Input: part model. Units: mm. Frame: model coordinates. A direction names the side the tool comes from. Coordinates: 2 decimals unless noted, no trailing zeros. Loops run counter-clockwise (first coordinate to the right, second up) from the corner with the lowest first, then second, coordinate; pieces in that order, holes last. Notation, with made-up numbers: (41, 31.25) -> (81, 31.25) arc R36 cw to (81, 67.25) -> close; hole circle Ø8 at (78.25, 70). An arc over 180 degrees is marked (long way). Put each result on its own line as item: value. Start each with the question number.
1) Material intervals for L1, parallel to X at y = 25, z = 58; L2, parallel to Y at x = 6, z = 56 (3 decimals); L3, parallel to X at y = -9.5, z = -5, sorted ascending.
2) Pull-direction query (X, two-part tool) for faces 1 (the flat face through (0, 11, 60.325)), 2 (the cylindrical face through (28.465, 14.972, 26.433)), 3 (the flat face through (-31.75, -1, 2)); classes: pulls with the +X half, pulls with the -X half, needs draft (parallel to the pull), parting line crosses it, or undercut.
3) Set-up query: faces 4 (the flat face through (-27, 15.875, -51)), 5 (the cylindrical face through (-28.63, 14.94, 26.3)), 6 (the cylindrical face through (0.493, 1.87, -52.925)). Return all of +Z, -Z, +X, -X, +Y, -Y with unobstructed straight access to the full face (end or side cutting, diameter ignored); none if empty.
4) Cut plane A-A (x = -6). Return the cut outline in (y, z) (3 decimals), plus the area to 3 significant figures.
5) Cut plane B-B (z = 36). Return the cut outline in (x, y) (3 decimals), plus the area to 3 significant figures.
6) Contact query for flat-ended pins moving along their axis: P1, Ø8, axis at x = -6.35, y = 25.4, coming from the -Z side (3 decimals); P2, Ø19, axis at x = 3, y = 26.5, coming from the -Z side; P3, Ø4, axis at x = 6.35, y = 25.4, coming from the +Z side; P4, Ø12, axis at x = -27.5, z = -47, coming from the +Y side (3 decimals). Output: stop coordinate, or through.
7) Cut plane D-D (y = 9). State how many separate pieces and enclosed holes the cut face has, plus the area to 3 significant figures.
8) Cut plane C-C (x = -28). Return the cut outline in (y, z) (1 decimal), plus the area to 3 significant figures.
from build123d import *

# Parameters (mm, degrees)
SKETCH1_W               = 107.95
SKETCH1_H               = 31.75
BOSS_EXTRUDE1_DEPTH     = 31.75
SKETCH3_W               = 63.5
SKETCH3_H               = 76.2
SKETCH3_R               = 3.429
BOSS_EXTRUDE2_DEPTH     = 6.35
FILLET1_R               = 5.08
CUT_EXTRUDE1_DEPTH      = 119.79762203
CUT_EXTRUDE1_DEPTH_BACK = 119.79762203
SKETCH4_W               = 78.111463513
SKETCH4_H               = 26.600111828


with BuildPart() as part:
    # Sketch1 → Boss-Extrude1 (new, symmetric)
    with BuildSketch(Plane(origin=(0, 0, 0), x_dir=(0, 0, -1), z_dir=(1, 0, 0))):
        Rectangle(SKETCH1_W, SKETCH1_H)
    extrude(amount=BOSS_EXTRUDE1_DEPTH, both=True)

    # Sketch2 → Cut-Revolve1 (revolve, cut)
    with BuildSketch(Plane(origin=(0, 0, 0), x_dir=(0, 0, -1), z_dir=(1, 0, 0))):
        Polygon((30.787113889, -1.024256513), (21.709471638, -34.902478605), (-1.905, -28.575), (15.934173595, 38.001702221), (59.482939473, 26.332845573), (50.721408129, -6.365634557), align=None)
    revolve(axis=Axis((0, -21.465443212, 0), (0, 0.9659258262890701, -0.2588190451025143)), mode=Mode.SUBTRACT)

    # Sketch3 → Boss-Extrude2 (add)
    with BuildSketch(Plane.XY.offset(53.975)):
        Rectangle(SKETCH3_W, SKETCH3_H)
        with Locations((-19.05, 25.4)):
            Circle(SKETCH3_R, mode=Mode.SUBTRACT)
        with Locations((-6.35, 25.4)):
            Circle(SKETCH3_R, mode=Mode.SUBTRACT)
        with Locations((6.35, 25.4)):
            Circle(SKETCH3_R, mode=Mode.SUBTRACT)
        with Locations((19.05, 25.4)):
            Circle(SKETCH3_R, mode=Mode.SUBTRACT)
        with Locations((-6.35, -25.4)):
            Circle(SKETCH3_R, mode=Mode.SUBTRACT)
        with Locations((6.35, -25.4)):
            Circle(SKETCH3_R, mode=Mode.SUBTRACT)
        with Locations((19.05, -25.4)):
            Circle(SKETCH3_R, mode=Mode.SUBTRACT)
        with Locations((-19.05, -25.4)):
            Circle(SKETCH3_R, mode=Mode.SUBTRACT)
    extrude(amount=BOSS_EXTRUDE2_DEPTH)

    # Fillet1
    fillet1_edges = [part.edges().sort_by_distance(p)[0] for p in [
        (0, 15.875, 53.975),
        (0, -15.875, 53.975),
    ]]
    fillet(fillet1_edges, radius=FILLET1_R)

    # Sketch4 → Cut-Extrude1 (cut, two sides: drawn at the far end of the back side and taken through both)
    with BuildSketch(Plane(origin=(0, 0, 53.975), x_dir=(-1, 0, 0), z_dir=(0, 0, -1)).offset(-CUT_EXTRUDE1_DEPTH_BACK)):
        with Locations((-0.534278136, -29.175055914)):
            Rectangle(SKETCH4_W, SKETCH4_H)
    extrude(amount=CUT_EXTRUDE1_DEPTH + CUT_EXTRUDE1_DEPTH_BACK, mode=Mode.SUBTRACT)


solid = part.part
Results found:
1. L1: x = -31.75 to -22.46, -15.64 to -9.76, -2.94 to 2.94, 9.76 to 15.64, 22.46 to 31.75
1. L2: y = -15.875 to 21.989, 28.811 to 38.1
1. L3: x = -31.75 to -24.39, 24.39 to 31.75
2. face 1: needs draft
2. face 2: undercut
2. face 3: pulls with the -X half
3. face 4: -Z, +X, -X, +Y
3. face 5: none
3. face 6: +Y
4. outline: (-15.875, -53.975) -> (7.326, -53.975) -> (-6.262, -50.334) -> (-0.831, -30.065) -> (-15.875, -26.034) -> close; (-15.875, 23.038) -> (11.437, 15.72) -> (15.875, 32.282) -> (15.875, 48.895) arc R5.08 cw to (20.955, 53.975) -> (21.989, 53.975) -> (21.989, 60.325) -> (-15.875, 60.325) -> close; (28.811, 53.975) -> (38.1, 53.975) -> (38.1, 60.325) -> (28.811, 60.325) -> close
4. area: 1,720 mm2
5. outline: (-31.75, -15.875) -> (31.75, -15.875) -> (31.75, 15.875) -> (-31.75, 15.875) -> close
5. area: 2,020 mm2
6. P1: stops at z = 53.975
6. P2: stops at z = 52.08
6. P3: passes through
6. P4: stops at y = 15.875
7. separate pieces: 3
7. enclosed holes: 0
7. area: 3,340 mm2
8. outline: (-15.9, -54) -> (15.9, -54) -> (15.9, -46.6) -> (-3.8, -41.3) -> (14.4, 27) -> (15.9, 26.6) -> (15.9, 48.9) arc R5.1 cw to (21, 54) -> (38.1, 54) -> (38.1, 60.3) -> (-15.9, 60.3) -> close
8. area: 3,000 mm2
